Geometry check sheet. Reference: the model listing, model coordinates, mm. A direction names the side the tool comes from. Give positions to 0.01 mm unless a question says otherwise; leave off trailing zeros. Order: outer loops, then holes, each group sorted by start corner. A loop starts at its lowest first (then second) coordinate and runs counter-clockwise, first axis right, second up.
```python
from build123d import *

# Parameters (mm, degrees)
SKETCH_1_R          = 5
EXTRUDE_1_DEPTH     = 7.5
SKETCH_2_W          = 6
SKETCH_2_H          = 15
EXTRUDE_2_DEPTH     = 15
FILLET_1_R          = 7.5
SKETCH_3_W          = 2
SKETCH_3_H          = 15
CUT_EXTRUDE_1_DEPTH = 44.603325561
SKETCH_4_R          = 2
CUT_EXTRUDE_2_DEPTH = 15
SKETCH_7_R          = 2.5
CUT_EXTRUDE_3_DEPTH = 40.714606885


with BuildPart() as part:
    # 草图1 → 凸台-拉伸1 (new, symmetric)
    with BuildSketch(Plane.XY):
        with BuildLine():
            Line((-26.031373033, 4.5), (26.031373033, 4.5))
            ThreePointArc((26.031373033, 4.5), (36, 0), (26.031373033, -4.5))
            Line((26.031373033, -4.5), (-26.031373033, -4.5))
            ThreePointArc((-26.031373033, -4.5), (-36, 0), (-26.031373033, 4.5))
        make_face()
        with Locations((-30, 0)):
            Circle(SKETCH_1_R, mode=Mode.SUBTRACT)
        with Locations((30, 0)):
            Circle(SKETCH_1_R, mode=Mode.SUBTRACT)
    extrude(amount=EXTRUDE_1_DEPTH, both=True)

    # 草图2 → 凸台-拉伸2 (add)
    with BuildSketch(Plane.XY.offset(7.5)):
        with Locations((0, 12)):
            Rectangle(SKETCH_2_W, SKETCH_2_H)
    extrude(amount=-EXTRUDE_2_DEPTH)

    # 圆角1
    fillet_1_edges = [part.edges().sort_by_distance(p)[0] for p in [
        (0, 19.5, 7.5),
        (0, 19.5, -7.5),
    ]]
    fillet(fillet_1_edges, radius=FILLET_1_R - 0.0001)  # a hair under: the kernel refuses the full size

    # 草图3 → 切除-拉伸1 (cut, through all)
    with BuildSketch(Plane.XY.offset(7.5)):
        with Locations((0, 12)):
            Rectangle(SKETCH_3_W, SKETCH_3_H)
    extrude(amount=-CUT_EXTRUDE_1_DEPTH, mode=Mode.SUBTRACT)

    # 草图4 → 切除-拉伸2 (cut)
    with BuildSketch(Plane.ZY.offset(3)):
        with Locations(Location((0, 12, 0), (0, 0, 270))):
            Circle(SKETCH_4_R)
    extrude(amount=-CUT_EXTRUDE_2_DEPTH, mode=Mode.SUBTRACT)

    # 草图7 → 切除-拉伸3 (cut, through all)
    with BuildSketch(Plane(origin=(0, 4.5, 0), x_dir=(1, 0, 0), z_dir=(0, 1, 0))):
        with Locations(Location((-15, 0, 0), (0, 0, 270))):
            Circle(SKETCH_7_R)
        with Locations(Location((15, 0, 0), (0, 0, 270))):
            Circle(SKETCH_7_R)
    extrude(amount=-CUT_EXTRUDE_3_DEPTH, mode=Mode.SUBTRACT)


solid = part.part
```
Q1. Thickness scan on L1, parallel to X at y = 13.5, z = -6; L2, parallel to Y at x = 30, z = 4.25; L3, parallel to X at y = -3.5, z = -2.25. Record the ranges inside material, lowest first.
Q2. Cross-section at D-D, the plane z = -0.75. Give the number of separate pieces and of enclosed holes in the cut face, and give its area (4 significant figures).
Q3. Access from +Z, -Z, +X, -X, +Y, -Y to the whole of each face (thin tool, end or side, straight path). Record for faces 1 (the face through (2.014, 17.245, -5.361)), 2 (the face through (-1, 10, -2)), 3 (the face through (0, -4.5, 0)).
Q4. Release check for a two-part mould opening along Y. For faces 4 (the face through (0, 4.5, 0)), 5 (the face through (-35, 0, 0)), 6 (the face through (-3, 10, -2)) record: pulls with the +Y half, pulls with the -Y half, needs draft (parallel to the pull), parting line crosses it, or undercut.
Q5. Cross-section at A-A, the plane y = 0. Record the boundary of the cut face in (x, z), and give its area (3 significant figures).
Q6. Cross-section at B-B, the plane x = 30. Record the boundary of the cut face in (y, z).
Q7. Gauge pin test, flat ends, axial feed: P1, Ø6.5, axis at x = 15, z = 0, coming from the -Y side; P2, Ø0.6, axis at x = 0, z = 0.5, coming from the +Y side; P3, Ø7.5, axis at y = 11.5, z = 0, coming from the +X side. Record the tip position at first contact, or that the pin passes through.
Q8. Cross-section at C-C, the plane y = 6.75. Record the boundary of the cut face in (x, z), and give its area (3 significant figures).
Answers follow:
1. L1: x = -3 to -1, 1 to 3
1. L2: y = -6 to -5, 5 to 6
1. L3: x = -34.87 to -33.57, -26.43 to -16.09, -13.91 to 13.91, 16.09 to 26.43, 33.57 to 34.87
2. separate pieces: 5
2. enclosed holes: 2
2. area: 471.5 mm2
3. face 1: -Z, +X, -X, +Y
3. face 2: +Z, -Z, +Y
3. face 3: +Z, -Z, -Y
4. face 4: pulls with the +Y half
4. face 5: undercut
4. face 6: needs draft
5. outline: (-36, -7.5) - (-35, -7.5) - (-35, 7.5) - (-36, 7.5) - close; (-25, -7.5) - (25, -7.5) - (25, 7.5) - (-25, 7.5) - close; (35, -7.5) - (36, -7.5) - (36, 7.5) - (35, 7.5) - close; hole circle Ø5 at (-15, 0); hole circle Ø5 at (15, 0)
5. area: 741 mm2
6. outline: (-6, -7.5) - (-5, -7.5) - (-5, 7.5) - (-6, 7.5) - close; (5, -7.5) - (6, -7.5) - (6, 7.5) - (5, 7.5) - close
7. P1: stops at y = -4.5
7. P2: stops at y = 4.5
7. P3: stops at x = 3
8. outline: (-3, -7.5) - (-1, -7.5) - (-1, 7.5) - (-3, 7.5) - close; (1, -7.5) - (3, -7.5) - (3, 7.5) - (1, 7.5) - close
8. area: 60.0 mm2
